from build123d import *

# Parameters (mm, degrees)
BOSS_EXTRUDE4_START   = 53.880055185
BOSS_EXTRUDE4_2_DEPTH = 71.319944815
BOSS_EXTRUDE4_START_2 = 52.05
BOSS_EXTRUDE4_3_DEPTH = 4.040129852
SKETCH26_R            = 8.2
BOSS_EXTRUDE5_DEPTH   = 1.5
FILLET8_R             = 0.25
FILLET9_R             = 0.4
FILLET10_R            = 0.5


with BuildPart() as part:
    # Boss-Extrude4: read off the stored shape, not the designer's step
    # Boss-Extrude4 outline → Boss-Extrude4 (revolve)
    with BuildSketch(Plane.YX):
        with BuildLine():
            Line((0, 52.05), (0, 50.45))
            add(Edge.make_bspline(
                [(6.25, 51.15), (3.15111586, 50.566822676), (0, 50.45)],
                knots=[1.384782418, 1.384782418, 1.384782418, 1.533739867, 1.533739867, 1.533739867], degree=2, weights=[1, 0.997227742, 1]))
            Line((6.25, 51.15), (6.25, 52.05))
            Line((6.25, 52.05), (0, 52.05))
        make_face()
    revolve(axis=Axis((0, 0, 0), (1, 0, 0)))



with BuildPart() as body_2:
    # Boss-Extrude4 2 outline → Boss-Extrude4 2 (new body)
    with BuildSketch(Plane.YZ.offset(BOSS_EXTRUDE4_START)):
        with BuildLine():
            Line((-0.496702112, -0.496702112), (-0.40023184, -6.023480263))
            ThreePointArc((-0.40023184, -6.023480263), (0, -6.036762377), (0.40023184, -6.023480263))
            Line((0.40023184, -6.023480263), (0.496702112, -0.496702112))
            Line((0.496702112, -0.496702112), (6.023480263, -0.40023184))
            ThreePointArc((6.023480263, -0.40023184), (6.036762377, 0), (6.023480263, 0.40023184))
            Line((6.023480263, 0.40023184), (0.496702112, 0.496702112))
            Line((0.496702112, 0.496702112), (0.40023184, 6.023480263))
            ThreePointArc((0.40023184, 6.023480263), (0, 6.036762377), (-0.40023184, 6.023480263))
            Line((-0.40023184, 6.023480263), (-0.496702112, 0.496702112))
            Line((-0.496702112, 0.496702112), (-6.023480263, 0.40023184))
            ThreePointArc((-6.023480263, 0.40023184), (-6.036762377, 0), (-6.023480263, -0.40023184))
            Line((-6.023480263, -0.40023184), (-0.496702112, -0.496702112))
        make_face()
    extrude(amount=BOSS_EXTRUDE4_2_DEPTH)


with BuildPart() as part_1:
    add(part.part)

    add(body_2.part)  # Boss-Extrude4 3 merges body 2
    # Boss-Extrude4 3 outline → Boss-Extrude4 3 (add)
    with BuildSketch(Plane.YZ.offset(BOSS_EXTRUDE4_START_2)):
        with BuildLine():
            Line((-4.58028551, -0.425422898), (-0.496702112, -0.496702112))
            Line((-0.496702112, -0.496702112), (-0.425422898, -4.58028551))
            ThreePointArc((-0.425422898, -4.58028551), (0, -4.6), (0.425422898, -4.58028551))
            Line((0.425422898, -4.58028551), (0.496702112, -0.496702112))
            Line((0.496702112, -0.496702112), (4.58028551, -0.425422898))
            ThreePointArc((4.58028551, -0.425422898), (4.6, 0), (4.58028551, 0.425422898))
            Line((4.58028551, 0.425422898), (0.496702112, 0.496702112))
            Line((0.496702112, 0.496702112), (0.425422898, 4.58028551))
            ThreePointArc((0.425422898, 4.58028551), (0, 4.6), (-0.425422898, 4.58028551))
            Line((-0.425422898, 4.58028551), (-0.496702112, 0.496702112))
            Line((-0.496702112, 0.496702112), (-4.58028551, 0.425422898))
            ThreePointArc((-4.58028551, 0.425422898), (-4.6, 0), (-4.58028551, -0.425422898))
        make_face()
    extrude(amount=BOSS_EXTRUDE4_3_DEPTH)

    # Boss-Extrude4 4 outline → Boss-Extrude4 4 (revolve, cut)
    with BuildSketch(Plane.YX):
        with BuildLine():
            Line((6.036762378, 53.880055185), (6.036762377, 56.090129852))
            ThreePointArc((6.036762377, 56.090129852), (5.645999412, 54.772109014), (4.6, 53.880055286))
            Line((4.6, 53.880055286), (6.036762378, 53.880055185))
        make_face()
    revolve(axis=Axis((0, 0, 0), (1, 0, 0)), mode=Mode.SUBTRACT)

    # Sketch26 → Boss-Extrude5 (add)
    with BuildSketch(Plane.ZY.offset(-125.2)):
        Circle(SKETCH26_R)
    extrude(amount=-BOSS_EXTRUDE5_DEPTH)

    # Fillet8
    fillet8_edges = [part_1.edges().sort_by_distance(p)[0] for p in [
        (89.540027592, 0.496702112, -0.496702112),
        (89.540027592, -0.496702112, -0.496702112),
        (89.540027592, -0.496702112, 0.496702112),
        (89.540027592, 0.496702112, 0.496702112),
    ]]
    fillet(fillet8_edges, radius=FILLET8_R)

    # Fillet9
    fillet9_edges = [part_1.edges().sort_by_distance(p)[0] for p in [
        (51.15, -6.25, 0),
    ]]
    fillet(fillet9_edges, radius=FILLET9_R)

    # Fillet10
    fillet10_edges = [part_1.edges().sort_by_distance(p)[0] for p in [
        (126.7, 0, -8.2),
        (125.2, 0, -8.2),
    ]]
    fillet(fillet10_edges, radius=FILLET10_R)


solid = part_1.part
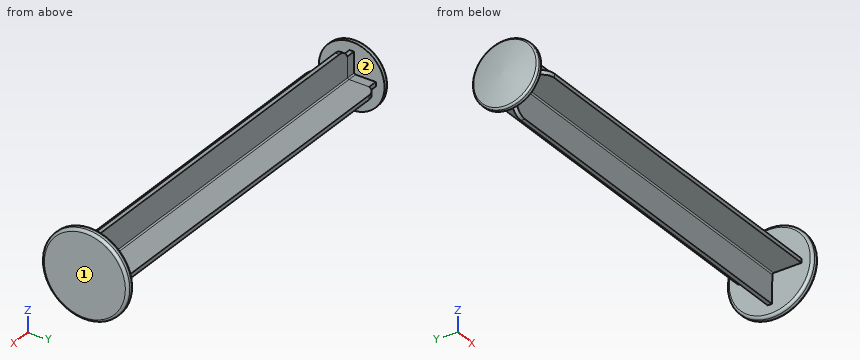
The model under review builds one solid part; all positions refer to its coordinate system, in mm. Face numbers are marked on the shaded views. Give positions to 0.01 mm unless a question says otherwise; leave off trailing zeros. Order: outer loops, then holes, each group sorted by start corner. A loop starts at its lowest first (then second) coordinate and runs counter-clockwise, first axis right, second up. Notation, with made-up numbers: (72.25, -33) -> (87.25, -33) arc R23 ccw to (87.25, -11) -> close; hole circle Ø7 at (56.25, -24). An arc over 180 degrees is marked (long way). Write item = value, one per line. Start each with the question number.
(1) Take a section at A-A (x = 60). Write out the cut boundary in (y, z), plus the area to 3 significant figures.
(2) Draft analysis for pull direction X (two halves, no side actions). For the marked faces 1 and 2, state which applies: +X half, -X half, draft (parallel to the pull), parting line (faces both ways), or undercut.
(3) For L1, parallel to X at y = 1.25, z = 5.75; L2, parallel to Z at x = 94, y = -1.25; L3, parallel to X at y = 1.5, z = -2.5, list the stretches that pass through material, from the lowest coordinate up. Write a range as from..to.
(4) For pin 1 Ø2 at (x, y) = (93.5, 0.5) entering from -Z; pin 2 Ø8 at (x, z) = (109, 1.5) entering from -Y; pin 3 Ø8 at (x, y) = (80, -5.5) entering from -Z, all flat-tipped, find the tip position at first contact; note any pin that passes through.
Returned:
q1.outline = (-6.02, -0.4) -> (-0.74, -0.49) arc R0.25 cw to (-0.49, -0.74) -> (-0.4, -6.02) arc R6.04 ccw to (0.4, -6.02) -> (0.49, -0.74) arc R0.25 cw to (0.74, -0.49) -> (6.02, -0.4) arc R6.04 ccw to (6.02, 0.4) -> (0.74, 0.49) arc R0.25 cw to (0.49, 0.74) -> (0.4, 6.02) arc R6.04 ccw to (-0.4, 6.02) -> (-0.49, 0.74) arc R0.25 cw to (-0.74, 0.49) -> (-6.02, 0.4) arc R6.04 ccw to start
q1.area = 20.9 mm²
q2.face_1 = +X half
q2.face_2 = undercut
q3.L1 = 51.08..52.05, 125.2..126.7
q3.L2 = -0.48..0.48
q3.L3 = 50.66..52.05, 125.2..126.7
q4.pin_1 = -6.04
q4.pin_2 = -6.04
q4.pin_3 = -0.48
